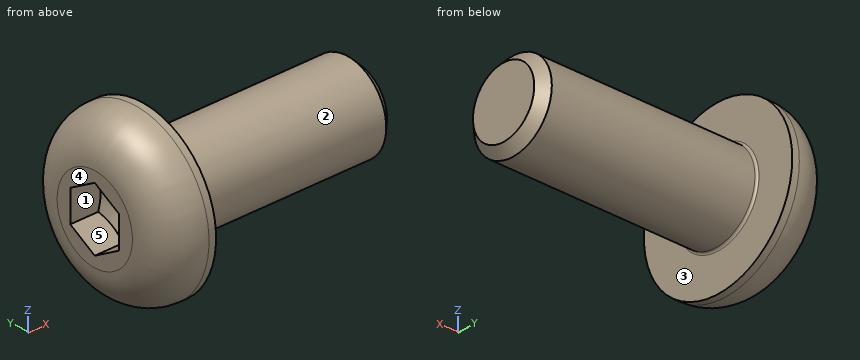
Autodesk Inventor part; units mm, degrees
ref_plane "Work Plane1" through (29, 0, 0) normal (0, -1, 0) x (1, 0, 0)
ref_plane "YZ Plane" through (0, 0, 0) normal (1, 0, 0) x (0, 1, 0)
ref_plane "XZ Plane" through (0, 0, 0) normal (0, 1, 0) x (-1, 0, 0)
sketch "Эскиз1" plane through (0, 0, 0) normal (0, 0, 1) x (1, 0, 0)
  line L0 (-0.0667, 0) -> (10, 0)
  line L1 (10, 0) -> (10, 2)
  line L2 (10, 2) -> (1.4, 2)
  line L3 (1.4, 2) -> (0.9705, 2)
  line L4 (0.9705, 2) -> (0, 2)
  line L5 (0, 2) -> (0, 3.8)
  line L6 (0, 3.8) -> (-2.2, 3.8)
  line L7 (-2.2, 3.8) -> (-2.2, 1.4434)
  line L8 (-2.2, 1.4434) -> (-0.9, 1.4434)
  line L9 (-0.9, 1.4434) -> (-0.0667, 0)
  line L10 (-4.64, 0) -> (12.44, 0)
  line L11 (0, -0.76) -> (0, 4.56)
  line L12 (1.4, 2) -> (0, 2) construction
  dimension "d1" = 8.6
  dimension "d2" = 0.4295
  dimension "d3" = 2.2
  dimension "d4" = 1.3
  dimension "d5" = 60
  dimension "d6" = 4
  dimension "d7" = 4
  dimension "d8" = 2.8868
  dimension "d9" = 7.6
  dimension "d26" = 10
revolve "Базовый элемент" add sketch "Эскиз1" angle 360 about axis through (-0.0667, 0, 0) along (1, 0, 0)
sketch "Эскиз2" plane through (-2.2, 0, 0) normal (-1, 0, 0) x (0, 0, 1)
  circle A0 centre (0, 0) radius 1.4434
  line L0 (0, -5.32) -> (0, 5.32)
  line L1 (-5.32, 0) -> (5.32, 0)
  line L2 (1.4434, 0) -> (0.7217, -1.25)
  line L3 (0.7217, -1.25) -> (-0.7217, -1.25)
  line L4 (-0.7217, -1.25) -> (-1.4434, 0)
  line L5 (-1.4434, 0) -> (-0.7217, 1.25)
  line L6 (-0.7217, 1.25) -> (0.7217, 1.25)
  line L7 (0.7217, 1.25) -> (1.4434, 0)
extrude "Паз" add sketch "Эскиз2" against normal up to next contours L7 A0 | A0 L2 | L6 L0 A0 | A0 L0 L3 | L0 L6 A0 | A0 L3 L0 | L4 A0 | A0 L5
fillet "Сопряжение1" radius 1.87 1 edges at (-2.2, -3.8, 0)
thread "Резьба"
chamfer "Фаска1" distance 0.4294 distance2 0.4294 1 edges at (10, -2, 0) measured on face at (10, 0.556, 0.0273)
ref_plane "Work Plane1" through (29, 0, 0) normal (0, -1, 0) x (1, 0, 0)
fillet "Fillet2" radius 0.1 1 edges at (0, -2, 0)
equation "\"d1\" = GEL"
equation "\"d3\" = KOH"
equation "\"d4\" = INTI"
equation "\"d6\" = GD"
equation "\"d7\" = BDM"
equation "\"d8\" = 1.1547 * SW"
equation "\"d9\" = KOD"
equation "\"d26\" = NLG"
equation "\"d30\" = R"
equation "\"d17\" = RR"
equation "\"d13\" = GEL"
equation "\"d15\" = -0.5 * SPD + 0.5 * GD"
equation "\"d16\" = GUL"
equation "\"GD\" = NND"
equation "\"NLG\" = 10"
equation "\"GEL\" = 8.6"
equation "\"KOD\" = 7.6"
equation "\"KOH\" = 2.2"
equation "\"INTI\" = 1.3"
equation "\"GAL\" = 0.61345 * PTC"
equation "\"GUL\" = 0.61345 * PTC"
equation "\"BDM\" = NND"
equation "\"SW\" = 2.5"
equation "\"RR\" = 1.87"
equation "\"SPD\" = 3.14117"
equation "\"R\" = 0.1"
equation "\"TOA\" = 30deg"
equation "\"GD1\" = THREADDIA - 1.2269 * PTC"
equation "\"THREADDIA\" = 4"
equation "\"PTC\" = 0.7"
equation "\"NND\" = 4"
equation "\"E0\" = 2.87"
properties part number "JIS B 1174 - M4 x 10" material "Сталь, мягкая"
Work out the finished part from the listing and answer in its coordinate system (mm). Face numbers are marked on the shaded views. A direction names the side the tool comes from. Give positions to 0.01 mm unless a question says otherwise; leave off trailing zeros. Loops run counter-clockwise (first coordinate to the right, second up) from the corner with the lowest first, then second, coordinate; pieces in that order, holes last. Notation, with made-up numbers: (-33, -6) -> (14, -6) arc R21 cw to (14, 32) -> close; hole circle Ø2 at (60.25, 5). An arc over 180 degrees is marked (long way). Use CSV: the item, a comma, the result in double quotes.
1. Flat-ended cylindrical pins translate along their axes: pin 1 Ø1.1 at (x, z) = (-1, 0) entering from +Y; pin 2 Ø3 at (x, z) = (5.5, 1) entering from -Y; pin 3 Ø0.7 at (x, z) = (-2, 0) entering from -Y. Find the tip coordinate at first contact, or state that the pin passes through.
Found:
pin 1,"y = 3.8"
pin 2,"y = -2"
pin 3,"y = -3.25"
2. The mould has two halves that part along Y. Classify the marked faces 1, 2 and 3: +Y half, -Y half, draft (parallel to the pull), parting line (faces both ways), or undercut.
Found:
face 1,"undercut"
face 2,"parting line"
face 3,"draft"
3. Straight lines are drawn through the part: line 1 (X direction, y = 0.5, z = 0.75); line 2 (X direction, y = 1, z = -2.25); line 3 (Z direction, x = 7.5, y = 1.75). For each, find the intervals that lie inside material, in ascending order.
Found:
line 1,"-0.59 to 10"
line 2,"-2.12 to 0"
line 3,"-0.97 to 0.97"
4. The part is cut by section A-A (x = 5.75). Write down the section's boundary in (y, z).
Found:
outline,"circle Ø4 at (0, 0)"
5. A tool of negligible diameter and unlimited length cuts with its end or side. For the marked faces 4 and 5, from which of +Z, -Z, +X, -X, +Y, -Y can it reach the whole face along a straight path? Write none if from no direction.
Found:
face 4,"+Z, -Z, -X, +Y, -Y"
face 5,"-X"
